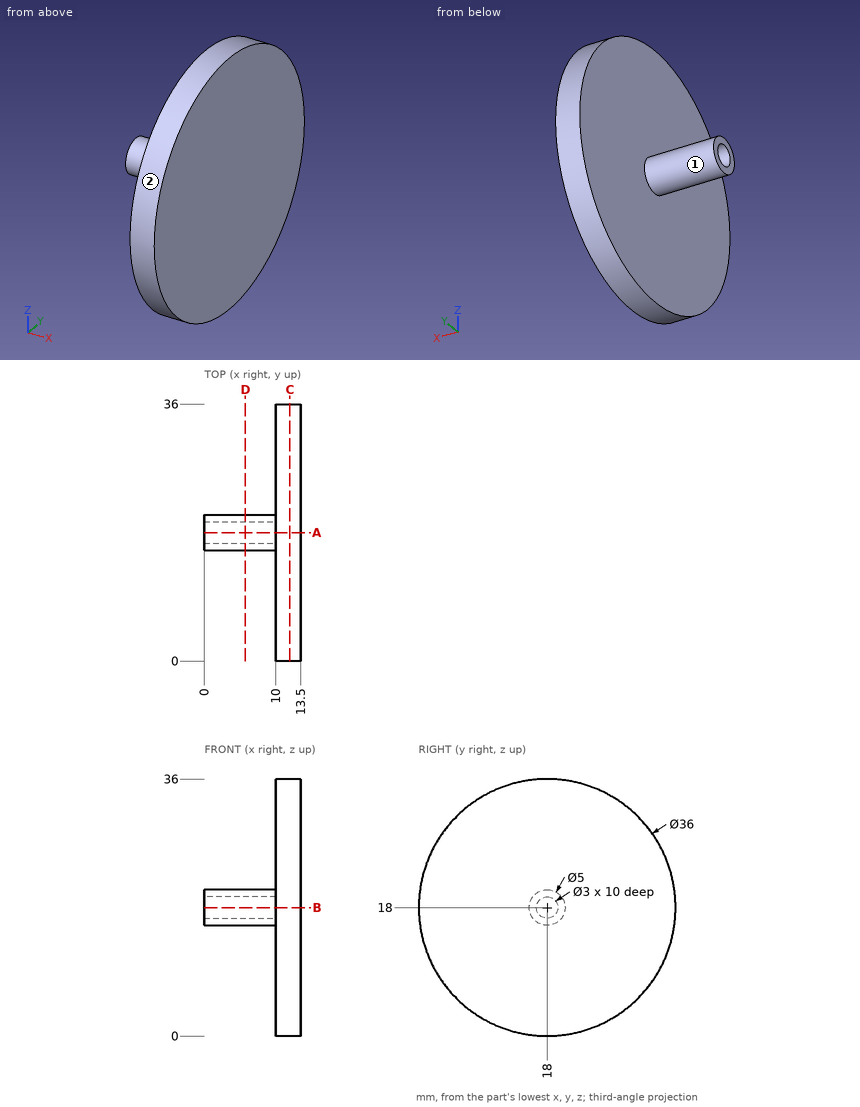
Could you check a few things on this drawing? It's one solid part, dimensions in mm from its lowest x, y, z. A direction names the side the tool comes from. Give positions to 0.01 mm unless a question says otherwise; leave off trailing zeros. Write each loop counter-clockwise with the first axis right and the second up, starting at its lowest first coordinate (ties: lowest second). Pieces come first, ordered by that corner, then holes.
(1) Imagine slicing it at D-D, the plane x = 5.75. Write out the boundary of the cut face in (y, z).
Output values:
outline: circle Ø5 at (18, 18); hole circle Ø3 at (18, 18)
(2) On a 3-axis mill with a long thin cutter (end or side, diameter ignored), from which of +Z, -Z, +X, -X, +Y, -Y can I reach the whole of each face in a straight line? I mean the marked faces 1 and 2. Say none if no direction works.
Output values:
face 1: -X
face 2: +X, -X
(3) If I drill on L1, parallel to Y at x = 7.5, z = 18; L2, parallel to X at y = 32.5, z = 22.5; L3, parallel to Y at x = 3.25, z = 17, over which ranges is the centre line in solid material (lowest first)?
Output values:
L1: y = 15.5 to 16.5, 19.5 to 20.5
L2: x = 10 to 13.5
L3: y = 15.71 to 16.88, 19.12 to 20.29
(4) Will these pins go through, and if not, where does the flat tip stop? pin 1 (2 mm diameter, centred on x = 11.5, y = 31.5, fed in from -Z); pin 2 (3 mm diameter, centred on x = 11.5, y = 16, fed in from -Z); pin 3 (5 mm diameter, centred on x = 9.5, z = 4.5, fed in from -Y).
Output values:
pin 1: stops at z = 5.05
pin 2: stops at z = 0.01
pin 3: stops at y = 3.79
(5) Imagine slicing it at C-C, the plane x = 12. Write out the boundary of the cut face in (y, z), and give its area (3 significant figures).
Output values:
outline: circle Ø36 at (18, 18)
area: 1,020 mm2
(6) Imagine slicing it at A-A, the plane y = 18. Write out the boundary of the cut face in (x, z), and give its area (3 significant figures).
Output values:
outline: (0, 15.5) - (10, 15.5) - (10, 0) - (13.5, 0) - (13.5, 36) - (10, 36) - (10, 20.5) - (0, 20.5) - (0, 19.5) - (10, 19.5) - (10, 16.5) - (0, 16.5) - close
area: 146 mm2
